Design review of the part shown in the three views and the two pictorial views. Dimensions are in mm from the part's minimum x, y and z. Coordinates: 2 decimals unless noted, no trailing zeros. Write each question's results on one line, items separated by ' | '.
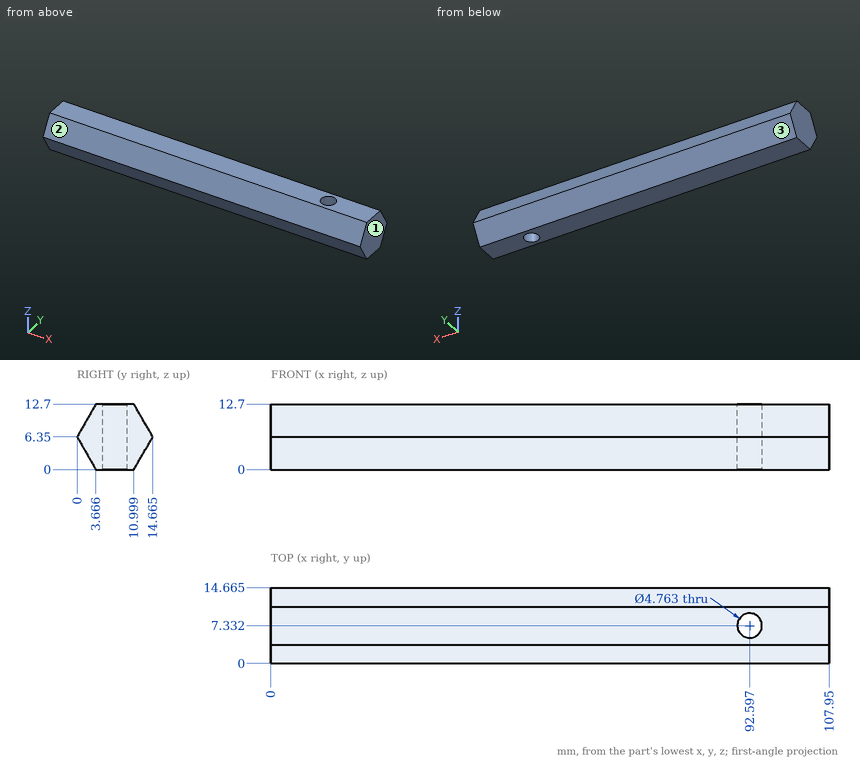
Q1. Mouldability with a two-part tool opening along Z and no side actions: class the marked faces 1, 2 and 3 as pulls with the +Z half, pulls with the -Z half, needs draft (parallel to the pull), parting line crosses it, or undercut.
Results found:
face 1: needs draft | face 2: pulls with the +Z half | face 3: pulls with the -Z half
Q2. Wall thickness on line 1 along X through (y, z) = (7.25, 4); line 2 along Y through (x, z) = (63.5, 6); line 3 along Y through (x, z) = (88.5, 12): over which ranges is each line inside the solid? List them lowest first. Write a range as from..to.
Results found:
line 1: 0..90.22, 94.98..107.95 | line 2: 0.2..14.46 | line 3: 3.26..11.4
Q3. For pin 1 (2 mm diameter, centred on x = 84, z = 8.5, fed in from -Y) (1 decimal); pin 2 (1 mm diameter, centred on x = 31, y = 3, fed in from +Z) (1 decimal); pin 3 (6 mm diameter, centred on x = 88.5, z = 11, fed in from +Y); pin 4 (3 mm diameter, centred on x = 92.6, y = 7.33, fed in from +Z), all flat-tipped, find the tip position at first contact; note any pin that passes through.
Results found:
pin 1: y = 0.7 | pin 2: z = 12.4 | pin 3: y = 13.71 | pin 4: through
